from build123d import *

# Parameters (mm, degrees)
SKETCH1_W          = 5
SKETCH1_H          = 75
SKETCH2_W          = 2.25
SKETCH2_H          = 2.25
CUT_EXTRUDE1_DEPTH = 10
CHAMFER1_SIZE      = 0.2


with BuildPart() as part:
    # Sketch1 → Revolve1 (revolve)
    with BuildSketch(Plane.XY, mode=Mode.PRIVATE) as revolve1_sk:
        with Locations((2.5, 37.5)):
            Rectangle(SKETCH1_W, SKETCH1_H)
    revolve(revolve1_sk.sketch.rotate(Axis((0, 75, 0), (0, -1, 0)), 180), axis=Axis((0, 75, 0), (0, -1, 0)))

    # Sketch2 → Cut-Extrude1 (cut)
    with BuildSketch(Plane.XZ):
        with Locations((0, 5)):
            Rectangle(SKETCH2_W, SKETCH2_H)
    extrude(amount=-CUT_EXTRUDE1_DEPTH, mode=Mode.SUBTRACT)

    # Chamfer1
    chamfer1_edges = [part.edges().sort_by_distance(p)[0] for p in [
        (1.125, 0, 4.373396909),
        (0, 0, 3.875),
        (5, 75, 0),
        (3.112474899, 0, -3.913118961),
        (-1.125, 0, 4.373396909),
    ]]
    chamfer(chamfer1_edges, length=CHAMFER1_SIZE)


solid = part.part
For this review, take the finished solid that the model builds, in its own axes (mm). A direction names the side the tool comes from. Round coordinates to 2 decimals unless told otherwise and drop trailing zeros. Write each loop counter-clockwise with the first axis right and the second up, starting at its lowest first coordinate (ties: lowest second). Pieces come first, ordered by that corner, then holes. Notation, with made-up numbers: (77, 79.5) -> (114, 79.5) arc R16 ccw to (114, 85.5) -> close; hole circle Ø5 at (10.25, 46). An arc over 180 degrees is marked (long way). Use CSV: the item, a comma, the result in double quotes.
(1) Clearance check with flat-ended pins moving along their axes: P1, Ø1.5, axis at y = 18.5, z = 1.5, coming from the -X side; P2, Ø3, axis at x = 2, y = 27.5, coming from the +Z side; P3, Ø1, axis at x = 2.5, y = 36.5, coming from the +Z side. State where each tip first meets the part, or that it passes through.
Computed values:
P1,"x = -4.94"
P2,"z = 4.97"
P3,"z = 4.58"
(2) Consider section A-A, the plane x = 0. Give the boundary of the cut face in (y, z) (3 decimals).
Computed values:
outline,"(0, -4.8) -> (0.2, -5) -> (74.8, -5) -> (75, -4.8) -> (75, 4.8) -> (74.8, 5) -> (10, 5) -> (10, 3.875) -> (0.2, 3.875) -> (0, 3.675) -> close"
(3) To check wall thickness, follow L1, parallel to Y at x = 0.25, z = 4.25; L2, parallel to Z at x = 2, y = 23.5; L3, parallel to X at y = 44, z = 4. State the ranges of each line that lie inside material, in increasing order. Write a range as [from, to].
Computed values:
L1,"[10, 75]"
L2,"[-4.58, 4.58]"
L3,"[-3, 3]"
(4) For faces 1 (the face through (0, 5, 3.875)), 2 (the face through (0.651, 38.022, -4.957)), list the 3-axis set-ups (+Z, -Z, +X, -X, +Y, -Y) from which the entire face can be reached by the end or side of a thin tool; tool diameter is ignored.
Computed values:
face 1,"+Z, -Y"
face 2,"+Y, -Y"
(5) Consider section B-B, the plane y = 6.5. Give the boundary of the cut face in (x, z) (3 decimals), plus the area to 3 significant figures.
Computed values:
outline,"(-1.125, 3.875) -> (-1.125, 4.872) arc R5 ccw (long way) to (1.125, 4.872) -> (1.125, 3.875) -> close"
area,"76.1 mm²"
